from build123d import *

# Parameters (mm, degrees)
SKETCH_W     = 30
SKETCH_H     = 12
PAD_DEPTH    = 1
SKETCH001_R  = 2.75
PAD001_DEPTH = 4
POCKET_DEPTH = 4
FILLET_R     = 0.3
FILLET001_R  = 1


with BuildPart() as part:
    # Sketch → Pad (new body)
    with BuildSketch(Plane.XY):
        Rectangle(SKETCH_W, SKETCH_H)
    extrude(amount=PAD_DEPTH)

    # Sketch001 (on Face6 of Pad) → Pad001 (join)
    with BuildSketch(Plane.XY.offset(1)):
        Circle(SKETCH001_R)
        with Locations((-12, 0)):
            Circle(SKETCH001_R)
        with Locations((12, 0)):
            Circle(SKETCH001_R)
    extrude(amount=PAD001_DEPTH)

    # Sketch002 (on Face11 of Pad001) → Pocket (cut)
    with BuildSketch(Plane.XY.offset(5)):
        Polygon((-0.65, 2.05), (-0.65, 0.7), (-2.05, 0.7), (-2.05, -0.7), (-0.65, -0.7), (-0.65, -2.05), (0.65, -2.05), (0.65, -0.7), (2.05, -0.7), (2.05, 0.7), (0.65, 0.7), (0.65, 2.05), align=None)
        Polygon((11.35, 2.05), (11.35, 0.7), (9.95, 0.7), (9.95, -0.7), (11.35, -0.7), (11.35, -2.05), (12.65, -2.05), (12.65, -0.7), (14.05, -0.7), (14.05, 0.7), (12.65, 0.7), (12.65, 2.05), align=None)
        Polygon((-12.65, 2.05), (-12.65, 0.7), (-14.05, 0.7), (-14.05, -0.7), (-12.65, -0.7), (-12.65, -2.05), (-11.35, -2.05), (-11.35, -0.7), (-9.95, -0.7), (-9.95, 0.7), (-11.35, 0.7), (-11.35, 2.05), align=None)
    extrude(amount=-POCKET_DEPTH, mode=Mode.SUBTRACT)

    # Fillet
    fillet_edges = [part.edges().sort_by_distance(p)[0] for p in [
        (-0.65, 0.7, 3),
        (0.65, 0.7, 3),
        (-12.65, 0.7, 3),
        (-11.35, 0.7, 3),
        (11.35, 0.7, 3),
        (12.65, 0.7, 3),
        (12.65, -0.7, 3),
        (11.35, -0.7, 3),
        (0.65, -0.7, 3),
        (-0.65, -0.7, 3),
        (-11.35, -0.7, 3),
        (-12.65, -0.7, 3),
    ]]
    fillet(fillet_edges, radius=FILLET_R)

    # Fillet001
    fillet001_edges = [part.edges().sort_by_distance(p)[0] for p in [
        (-15, -6, 0.5),
        (15, -6, 0.5),
        (-15, 6, 0.5),
        (15, 6, 0.5),
    ]]
    fillet(fillet001_edges, radius=FILLET001_R)


solid = part.part
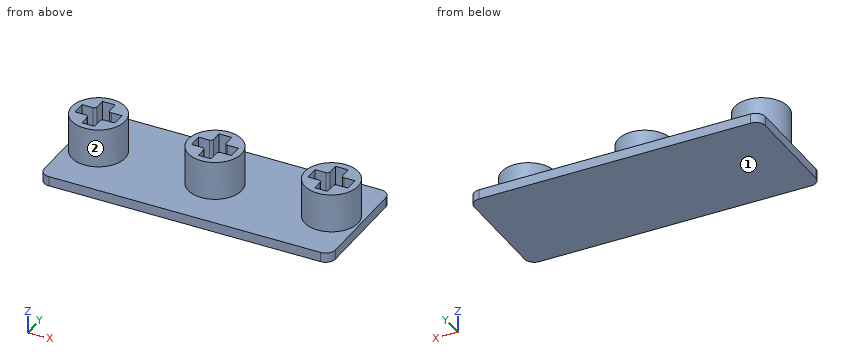
CAD build for the part. Positions are in the model's coordinates, mm. Face numbers are marked on the shaded views. Round coordinates to 2 decimals unless told otherwise and drop trailing zeros. Loops run counter-clockwise (first coordinate to the right, second up) from the corner with the lowest first, then second, coordinate; pieces in that order, holes last. Notation, with made-up numbers: M 25.5,-23.5 L 43.5,-23.5 A17 ccw 43.5,2.5 Z; hole C 69,-36 d3. An arc over 180 degrees is marked long. One line per question, with ' | ' between items. Start each with the question number.
Item 1: Wall check: line 1 (X direction, y = 0.5, z = 2.5); line 2 (X direction, y = -1.75, z = 3.25); line 3 (Y direction, x = 0, z = 4.85). Give the ranges that are in metal, low to high.
Item 2: Cut at D-D, the plane x = 8.75. Write the cut outline in (y, z).
Item 3: Cut at B-B, the plane z = 2.85. State how many separate pieces and enclosed holes the cut face has, plus the area to 3 significant figures.
Item 4: Pin check, flat tips, straight feed: pin 1 Ø0.5 at (x, z) = (-13.5, 4) entering from +Y; pin 2 Ø4 at (x, y) = (-2.5, 2.5) entering from -Z; pin 3 Ø1.1 at (y, z) = (-0.5, 3.5) entering from -X; pin 4 Ø2 at (x, z) = (2.5, 4.5) entering from +Y. Stop position of each tip, or through.
Item 5: Cut at C-C, the plane x = 0. Write the cut outline in (y, z).
Item 6: Two-plate mould, pull along X, no slides. Class the marked faces 1 and 2: pulls with the +X half, pulls with the -X half, needs draft (parallel to the pull), parting line crosses it, or undercut.
Item 7: Cut at A-A, the plane y = 0. Write the cut outline in (x, z), plus the area to 3 significant figures.
Responses:
1) line 1: x = -14.7 to -14.05, -9.95 to -9.3, -2.7 to -2.05, 2.05 to 2.7, 9.3 to 9.95, 14.05 to 14.7 | line 2: x = -14.12 to -12.65, -11.35 to -9.88, -2.12 to -0.65, 0.65 to 2.12, 9.88 to 11.35, 12.65 to 14.12 | line 3: y = -2.75 to -2.05, 2.05 to 2.75
2) outline: M -6,0 L 6,0 L 6,1 L -6,1 Z
3) separate pieces: 3 | enclosed holes: 3 | area: 43.3 mm²
4) pin 1: stops at y = 2.45 | pin 2: stops at z = 0 | pin 3: stops at x = -14.75 | pin 4: stops at y = 2.3
5) outline: M -6,0 L 6,0 L 6,1 L 2.75,1 L 2.75,5 L 2.05,5 L 2.05,1 L -2.05,1 L -2.05,5 L -2.75,5 L -2.75,1 L -6,1 Z
6) face 1: needs draft | face 2: undercut
7) outline: M -15,0 L 15,0 L 15,1 L 14.75,1 L 14.75,5 L 14.05,5 L 14.05,1 L 9.95,1 L 9.95,5 L 9.25,5 L 9.25,1 L 2.75,1 L 2.75,5 L 2.05,5 L 2.05,1 L -2.05,1 L -2.05,5 L -2.75,5 L -2.75,1 L -9.25,1 L -9.25,5 L -9.95,5 L -9.95,1 L -14.05,1 L -14.05,5 L -14.75,5 L -14.75,1 L -15,1 Z | area: 46.8 mm²
